from build123d import *

# Parameters (mm, degrees)
SKETCH1_W           = 18.5
SKETCH1_H           = 18.5
SKETCH1_W_2         = 14.5
SKETCH1_H_2         = 14.5
BOSS_EXTRUDE1_DEPTH = 60
SKETCH2_R           = 7.25
SKETCH2_R_2         = 5.25
BOSS_EXTRUDE2_DEPTH = 15
CHAMFER1_SIZE       = 5
CHAMFER1_SIZE_2     = 13.025445323


with BuildPart() as part:
    # Sketch1 → Boss-Extrude1 (new body)
    with BuildSketch(Plane(origin=(0, 0, 0), x_dir=(1, 0, 0), z_dir=(0, 1, 0))):
        Rectangle(SKETCH1_W, SKETCH1_H)
        Rectangle(SKETCH1_W_2, SKETCH1_H_2, mode=Mode.SUBTRACT)
    extrude(amount=BOSS_EXTRUDE1_DEPTH)

    # Sketch2 → Boss-Extrude2 (add)
    with BuildSketch(Plane.XY.offset(9.25)):
        with Locations(Location((0, 30, 0), (0, 0, 180))):
            Circle(SKETCH2_R)
        with Locations((0, 30)):
            Circle(SKETCH2_R_2, mode=Mode.SUBTRACT)
    extrude(amount=BOSS_EXTRUDE2_DEPTH)

    # Chamfer1
    # the kernel refuses this chamfer: 13.025445323, 5 mm, written as the material it adds along each edge
    with BuildSketch(Plane(origin=(0, 30, 9.25), x_dir=(-1, 0, 0), z_dir=(0, 1, 0))) as chamfer1_piece_1_section:
        Polygon((7.25 + CHAMFER1_SIZE, 0), (7.25, CHAMFER1_SIZE_2), (7.25, 0), align=None)
    chamfer1_piece_1 = revolve(axis=Axis((0, 30, 9.25), (0, 0, 1)), mode=Mode.PRIVATE)
    chamfer1_piece_1 = split(chamfer1_piece_1, bisect_by=Plane(origin=(-9.25, 20.104834993, 11.052414917), z_dir=(1, 0, 0)), keep=Keep.TOP, mode=Mode.PRIVATE)
    chamfer1_piece_1 = split(chamfer1_piece_1, bisect_by=Plane(origin=(9.25, 20.104834993, 11.052414917), z_dir=(-1, 0, 0)), keep=Keep.TOP, mode=Mode.PRIVATE)
    add(chamfer1_piece_1)


solid = part.part
Could you check a few things on this model? Use its own coordinates, in mm. A direction names the side the tool comes from. Round coordinates to 2 decimals unless told otherwise and drop trailing zeros. Order: outer loops, then holes, each group sorted by start corner. A loop starts at its lowest first (then second) coordinate and runs counter-clockwise, first axis right, second up. Notation, with made-up numbers: M -23,22 L -10,22 A12 ccw -10,27 Z; hole C -2,15.25 d3. An arc over 180 degrees is marked long. One line per item, written item: value.
(1) I need wall thicknesses on line 1 along Z through (x, y) = (3.5, 32); line 2 along Z through (x, y) = (-4.5, 34). Which ranges of each line are inside material? Lowest first, please. Write a range as from..to.
Ans:
line 1: z = -9.25..-7.25, 7.25..9.25
line 2: z = -9.25..-7.25, 7.25..24.25
(2) Which directions (+Z, -Z, +X, -X, +Y, -Y) give clear straight access to the entire face, cutting with the end or side of a thin tool? Please do faces 1 (the flat face through (7.25, 30, 0)), 2 (the flat face through (-9.25, 30, 1)), 3 (the cylindrical face through (-3.35, 36.43, 23.25)).
Ans:
face 1: +Y, -Y
face 2: +Z, -Z, -X, +Y, -Y
face 3: +Z
(3) I'm going to push flat-ended pins straight in: P1, Ø12, axis at y = 17, z = 12.5, coming from the +X side; P2, Ø9.5, axis at x = 4, y = 48, coming from the +Z side; P3, Ø8, axis at x = 6.5, z = 20, coming from the +Y side. Where does each tip first touch, or does it pass through?
Ans:
P1: stops at x = 9.25
P2: stops at z = 9.25
P3: stops at y = 38.45
(4) Imagine slicing it at D-D (y = 30). Write out the boundary of the cut face in (x, z).
Ans:
outline: M -9.25,-9.25 L 9.25,-9.25 L 9.25,17.07 L 7.25,22.28 L 7.25,24.25 L 5.25,24.25 L 5.25,9.25 L -5.25,9.25 L -5.25,24.25 L -7.25,24.25 L -7.25,22.28 L -9.25,17.07 Z; hole M -7.25,-7.25 L 7.25,-7.25 L 7.25,7.25 L -7.25,7.25 Z
(5) If we mould it in two halves opening along Z, with no side actions, what happens to faces 4 (the flat face through (0, 51, 9.25)), 5 (the flat face through (0, 30, 7.25)), 6 (the cylindrical face through (-0.683, 35.205, 16.645)), 7 (the flat face through (-7.25, 30, 0))? For each: released by +Z, released by -Z, zero draft, split by the parting line, or undercut.
Ans:
face 4: released by +Z
face 5: undercut
face 6: zero draft
face 7: undercut
(6) Imagine slicing it at A-A (x = 0). Write out the boundary of the cut face in (y, z).
Ans:
outline: M 0,-9.25 L 60,-9.25 L 60,-7.25 L 0,-7.25 Z; M 0,7.25 L 60,7.25 L 60,9.25 L 42.25,9.25 L 37.25,22.28 L 37.25,24.25 L 35.25,24.25 L 35.25,9.25 L 24.75,9.25 L 24.75,24.25 L 22.75,24.25 L 22.75,22.28 L 17.75,9.25 L 0,9.25 Z
(7) Imagine slicing it at C-C (y = 44). Write out the boundary of the cut face in (x, z), and give its area (3 significant figures).
Ans:
outline: M -9.25,-9.25 L 9.25,-9.25 L 9.25,9.25 L -9.25,9.25 Z; hole M -7.25,-7.25 L 7.25,-7.25 L 7.25,7.25 L -7.25,7.25 Z
area: 132 mm^2
(8) Imagine slicing it at B-B (z = -4.5). Write out the boundary of the cut face in (x, y), and give its area (3 significant figures).
Ans:
outline: M -9.25,0 L -7.25,0 L -7.25,60 L -9.25,60 Z; M 7.25,0 L 9.25,0 L 9.25,60 L 7.25,60 Z
area: 240 mm^2
